Could you check a few things on this model? Use its own coordinates, in mm. A direction names the side the tool comes from. Coordinates: 2 decimals unless noted, no trailing zeros. Write each loop counter-clockwise with the first axis right and the second up, starting at its lowest first coordinate (ties: lowest second). Pieces come first, ordered by that corner, then holes.
```python
from build123d import *

# Parameters (mm, degrees)
F2_DEPTH = 2.5
F3_W     = 2.5
F3_H     = 5
F4_DEPTH = 2
F5_W     = 2.5
F5_H     = 1
F6_W     = 2.5
F6_H     = 1
F7_DEPTH = 2
F8_SIZE  = 0.5


with BuildPart() as f2:
    # F1 (on Right) → F2 (new body)
    with BuildSketch(Plane.YZ):
        Polygon((0, 0), (40, 0), (40, 85.7802768204), align=None)
        Polygon((35, 5), (7.8484278856, 5), (35, 63.2267343021), align=None, mode=Mode.SUBTRACT)
    extrude(amount=F2_DEPTH)

    # F3 (on face) → F4 (join)
    with BuildSketch(Plane(origin=(0, 0, 0), x_dir=(1, 0, 0), z_dir=(0, -0.906307787, 0.4226182617))):
        with Locations((1.25, 62.1480633261)):
            Rectangle(F3_W, F3_H)
        with Locations((1.25, 37.1480633261)):
            Rectangle(F3_W, F3_H)
    extrude(amount=F4_DEPTH)

    # F5 (on face) + F6 (on face) → F7 (cut)
    with BuildSketch(Plane(origin=(0, 27.3214521478, 58.5910432093), x_dir=(1, 0, 0), z_dir=(0, 0.4226182617, 0.906307787))):
        with Locations((1.25, -0.5)):
            Rectangle(F5_W, F5_H)
    with BuildSketch(Plane(origin=(0, 16.7559956043, 35.9333485334), x_dir=(1, 0, 0), z_dir=(0, 0.4226182617, 0.906307787))):
        with Locations((1.25, -0.5)):
            Rectangle(F6_W, F6_H)
    extrude(amount=-F7_DEPTH, mode=Mode.SUBTRACT)

    # F8
    f8_edges = [f2.edges().sort_by_distance(p)[0] for p in [
        (1.25, 12.830289, 32.247046),
        (1.25, 23.395745, 54.904741),
    ]]
    chamfer(f8_edges, length=F8_SIZE)


solid = f2.part
```
1. I want a section at D-D on z = 65.5. Please give me the cut outline in (x, y).
Verdict:
outline: (0, 30.54) - (2.5, 30.54) - (2.5, 40) - (0, 40) - close
2. I want a section at A-A on x = 1.2. Please give me the cut outline in (y, z), plus the area to 3 significant figures.
Verdict:
outline: (0, 0) - (40, 0) - (40, 85.78) - (26.48, 56.78) - (25.57, 57.2) - (26.42, 59.01) - (25.51, 59.44) - (23.61, 55.36) - (23.85, 54.69) - (25.21, 54.06) - (15.91, 34.12) - (15, 34.54) - (15.85, 36.36) - (14.94, 36.78) - (13.04, 32.7) - (13.28, 32.04) - (14.64, 31.4) - close; hole (7.85, 5) - (35, 5) - (35, 63.23) - close
area: 941 mm2
3. If we mould it in two halves opening along Z, with no side actions, what happens to faces 1 (the face through (1, 20, 0)), 2 (the face through (1, 35, 35)), 3 (the face through (1, 40, 42)), 4 (the face through (1.233, 24.571, 57.426))? For each: pulls with the +Z half, pulls with the -Z half, needs draft (parallel to the pull), parting line crosses it, or undercut.
Verdict:
face 1: pulls with the -Z half
face 2: undercut
face 3: needs draft
face 4: pulls with the +Z half
4. I want a section at C-C on z = 22.5. Please give me the cut outline in (x, y), plus the area to 3 significant figures.
Verdict:
outline: (0, 10.49) - (2.5, 10.49) - (2.5, 16.01) - (0, 16.01) - close; (0, 35) - (2.5, 35) - (2.5, 40) - (0, 40) - close
area: 26.3 mm2
5. I want a section at B-B on y = 18. Please give me the cut outline in (x, z).
Verdict:
outline: (0, 0) - (2.5, 0) - (2.5, 5) - (0, 5) - close; (0, 26.77) - (2.5, 26.77) - (2.5, 38.6) - (0, 38.6) - close
6. Please list where these lines run through material, in increasing order: line 1 along Y through (x, z) = (2.2, 61.5); line 2 along Z through (x, y) = (2.3, 17.5); line 3 along Z through (x, y) = (1.9, 17).
Verdict:
line 1: y = 28.68 to 34.19, 35 to 40
line 2: z = 0 to 5, 25.7 to 37.53
line 3: z = 0 to 5, 24.63 to 36.46
7. On a 3-axis mill with a long thin cutter (end or side, diameter ignored), from which of +Z, -Z, +X, -X, +Y, -Y can I reach the whole of each face in a straight line? I mean faces 5 (the face through (1.23, 15.43, 35.46)), 6 (the face through (1.233, 14.006, 34.768)). Say none if no direction works.
Verdict:
face 5: +X, -X
face 6: +Z, +X, -X, -Y
8. For pin 1 (1.2 mm diameter, centred on x = 1.5, y = 23.5, fed in from +Z) (3 decimals); pin 2 (1.5 mm diameter, centred on x = 1, y = 9.5, fed in from +Z); pin 3 (0.8 mm diameter, centred on x = 1.5, z = 44, fed in from -Y), each with a flat end and sliding along its axis, tell me the tip position at first contact or that it passes through.
Verdict:
pin 1: stops at z = 56.415
pin 2: stops at z = 21.98
pin 3: stops at y = 20.33
